Check sheet for the modelled part. Datum: model origin and axes. Units: mm. A direction names the side the tool comes from. Coordinates: 2 decimals unless noted, no trailing zeros. Loops run counter-clockwise (first coordinate to the right, second up) from the corner with the lowest first, then second, coordinate; pieces in that order, holes last. Notation, with made-up numbers: (32.5, -26.5) - (44.5, -26.5) arc R26 ccw to (44.5, 5.5) - close; hole circle Ø10 at (-11, -27). An arc over 180 degrees is marked (long way). Answer as a JSON object with one key per item and string values. Group by question number.
from build123d import *

# Parameters (mm, degrees)
BOSS_EXTRUDE2_DEPTH = 2
BOSS_EXTRUDE4_DEPTH = 21
BOSS_EXTRUDE3_DEPTH = 20


with BuildPart() as part:
    # Sketch1 → Boss-Extrude2 (new body)
    with BuildSketch(Plane.XY):
        with BuildLine():
            Line((1.936491673, 0.5), (4.5, 0.5))
            Line((4.5, 0.5), (4.5, -0.5))
            Line((4.5, -0.5), (1.936491673, -0.5))
            ThreePointArc((1.936491673, -0.5), (0, -2), (-1.936491673, -0.5))
            Line((-1.936491673, -0.5), (-4.5, -0.5))
            Line((-4.5, -0.5), (-4.5, 0.5))
            Line((-4.5, 0.5), (-1.936491673, 0.5))
            ThreePointArc((-1.936491673, 0.5), (0, 2), (1.936491673, 0.5))
        make_face()
    extrude(amount=BOSS_EXTRUDE2_DEPTH)

    # Sketch2<2> → Boss-Extrude4 (add)
    with BuildSketch(Plane.XY.offset(2)):
        with BuildLine():
            Line((1.936491673, 0.5), (2.5, 0.5))
            Line((2.5, 0.5), (2.5, -0.5))
            Line((2.5, -0.5), (1.936491673, -0.5))
            ThreePointArc((1.936491673, -0.5), (0, -2), (-1.936491673, -0.5))
            Line((-1.936491673, -0.5), (-2.5, -0.5))
            Line((-2.5, -0.5), (-2.5, 0.5))
            Line((-2.5, 0.5), (-1.936491673, 0.5))
            ThreePointArc((-1.936491673, 0.5), (0, 2), (1.936491673, 0.5))
        make_face()
    extrude(amount=BOSS_EXTRUDE4_DEPTH)

    # Sketch2 → Boss-Extrude3 (add)
    with BuildSketch(Plane.XY.offset(2)):
        with BuildLine():
            Line((1.936491673, 0.5), (2.5, 0.5))
            Line((2.5, 0.5), (2.5, -0.5))
            Line((2.5, -0.5), (1.936491673, -0.5))
            ThreePointArc((1.936491673, -0.5), (0, -2), (-1.936491673, -0.5))
            Line((-1.936491673, -0.5), (-2.5, -0.5))
            Line((-2.5, -0.5), (-2.5, 0.5))
            Line((-2.5, 0.5), (-1.936491673, 0.5))
            ThreePointArc((-1.936491673, 0.5), (0, 2), (1.936491673, 0.5))
        make_face()
    extrude(amount=BOSS_EXTRUDE3_DEPTH)


solid = part.part
1. Sectioned sample at A-A on y = 0.15. Record the cut outline in (x, z).
2. Sectioned sample at C-C on x = 4. Record the cut outline in (y, z), plus the area to 3 significant figures.
3. Sectioned sample at D-D on y = -1.15. Record the cut outline in (x, z).
4. Gauge pin test, flat ends, axial feed: pin 1 (0.8 mm diameter, centred on x = -3.5, y = 0, fed in from +Z); pin 2 (1.1 mm diameter, centred on y = 0, z = 8.5, fed in from +X); pin 3 (0.8 mm diameter, centred on x = -2.5, z = 12.5, fed in from -Y); pin 4 (1 mm diameter, centred on x = -3.5, z = 14.5, fed in from +Y). Record the tip position at first contact, or that the pin passes through.
5. Sectioned sample at B-B on z = 8.75. Record the cut outline in (x, y).
6. Material ranges on line 1 (Y direction, x = 2.25, z = 2); line 2 (X direction, y = -0.25, z = 7); line 3 (Z direction, x = 3.5, y = -0.15), recorded low to high.
7. Access from +Z, -Z, +X, -X, +Y, -Y to the whole of each face (thin tool, end or side, straight path). Record for faces 1 (the face through (-2.2, 0.5, 8.9)), 2 (the face through (4, 0, 2)), 3 (the face through (-3, 0, 2)).
Answers follow:
{
 "1": {"outline": "(-4.5, 0) - (4.5, 0) - (4.5, 2) - (2.5, 2) - (2.5, 23) - (-2.5, 23) - (-2.5, 2) - (-4.5, 2) - close"},
 "2": {"outline": "(-0.5, 0) - (0.5, 0) - (0.5, 2) - (-0.5, 2) - close", "area": "2.00 mm^2"},
 "3": {"outline": "(-1.64, 0) - (1.64, 0) - (1.64, 23) - (-1.64, 23) - close"},
 "4": {"pin 1": "stops at z = 2", "pin 2": "stops at x = 2.5", "pin 3": "stops at y = -0.5", "pin 4": "passes through"},
 "5": {"outline": "(-2.5, -0.5) - (-1.94, -0.5) arc R2 ccw to (1.94, -0.5) - (2.5, -0.5) - (2.5, 0.5) - (1.94, 0.5) arc R2 ccw to (-1.94, 0.5) - (-2.5, 0.5) - close"},
 "6": {"line 1": "y = -0.5 to 0.5", "line 2": "x = -2.5 to 2.5", "line 3": "z = 0 to 2"},
 "7": {"face 1": "+Z, -Z, -X, +Y", "face 2": "+Z, +X, +Y, -Y", "face 3": "+Z, -X, +Y, -Y"}
}
